from build123d import *

# Parameters (mm, degrees)
SKETCH_1_R               = 246.95
SKETCH_1_R_2             = 223.5
EXTRUDE_5_DEPTH          = 22.45
SKETCH_1_5_R             = 5.6125
CUT_EXTRUDE_1_DEPTH      = 350.960865669
PATTERN_CIRCULAR_2_COUNT = 10


with BuildPart() as part:
    # Эскиз1 → Бобышка-Вытянуть5 (new body)
    with BuildSketch(Plane(origin=(0, 0, 0), x_dir=(1, 0, 0), z_dir=(0, 1, 0))):
        with Locations(Location((0, 0, 0), (0, 0, 270))):
            Circle(SKETCH_1_R)
        with Locations(Location((0, 0, 0), (0, 0, 270))):
            Circle(SKETCH_1_R_2, mode=Mode.SUBTRACT)
    extrude(amount=EXTRUDE_5_DEPTH)

    # Эскиз1<5> → Вырез-Вытянуть1 (cut, through all)
    with BuildSketch(Plane(origin=(0, 0, 0), x_dir=(1, 0, 0), z_dir=(0, 1, 0))):
        with Locations(Location((0, -235.225, 0), (0, 0, 270))):
            Circle(SKETCH_1_5_R)
    cut_extrude_1 = extrude(amount=CUT_EXTRUDE_1_DEPTH, mode=Mode.SUBTRACT)

    # Круговой массив2: Вырез-Вытянуть1 ×10 about axis
    pattern_circular_2_axis = Axis((0, 0, 0), (0, 1, 0))
    for i in range(1, PATTERN_CIRCULAR_2_COUNT):
        add(cut_extrude_1.rotate(pattern_circular_2_axis, i * 360 / PATTERN_CIRCULAR_2_COUNT), mode=Mode.SUBTRACT)


solid = part.part
The listing builds one solid part. Answer for the finished solid, in the listing's coordinates (mm). Coordinates: 2 decimals unless noted, no trailing zeros. Write each loop counter-clockwise with the first axis right and the second up, starting at its lowest first coordinate (ties: lowest second). Pieces come first, ordered by that corner, then holes. Notation, with made-up numbers: (1, 58) - (27, 58) arc R9 ccw to (27, 70) - close; hole circle Ø6 at (16.5, 24.25). An arc over 180 degrees is marked (long way). Return JSON: item names as keys, results as strings.
1. The part is cut by section A-A on z = 0. Determine the outline of the cut face in (x, y), then the cut area to 3 significant figures.
Final values:
{"outline": "(-246.95, 0) - (-223.5, 0) - (-223.5, 22.45) - (-246.95, 22.45) - close; (223.5, 0) - (246.95, 0) - (246.95, 22.45) - (223.5, 22.45) - close", "area": "1,050 mm^2"}
2. The part is cut by section B-B on x = 0. Determine the outline of the cut face in (y, z), then the cut area to 3 significant figures.
Final values:
{"outline": "(0, -246.95) - (22.45, -246.95) - (22.45, -240.84) - (0, -240.84) - close; (0, -229.61) - (22.45, -229.61) - (22.45, -223.5) - (0, -223.5) - close; (0, 223.5) - (22.45, 223.5) - (22.45, 229.61) - (0, 229.61) - close; (0, 240.84) - (22.45, 240.84) - (22.45, 246.95) - (0, 246.95) - close", "area": "549 mm^2"}
3. For a pull along X with two mould halves and no side action, classify faces 1 (the face through (166.901, 11.068, -182.012)), 2 (the face through (1.686, 11.068, 240.578)), 3 (the face through (38, 22.45, -221)), 4 (the face through (-140.045, 11.068, 195.623)) as +X half, -X half, draft (parallel to the pull), parting line (faces both ways), or undercut.
Final values:
{"face 1": "parting line", "face 2": "undercut", "face 3": "draft", "face 4": "undercut"}
4. Each of these flat-tipped pins is pushed along its axis until it touches: pin 1 Ø9 at (x, z) = (0, -235.225) entering from -Y; pin 2 Ø2 at (y, z) = (2.5, -190) entering from -X; pin 3 Ø2 at (y, z) = (15, -180) entering from +X; pin 4 Ø12 at (x, y) = (-82.5, 13.5) entering from +Z. Where does it stop, or does it pass through?
Final values:
{"pin 1": "through", "pin 2": "x = -158.94", "pin 3": "x = 170.13", "pin 4": "z = 234.8"}
5. The part is cut by section D-D on y = 16. Count the separate pieces of the cut face and the enclosed holes in it, then the cut area to 3 significant figures.
Final values:
{"separate pieces": "1", "enclosed holes": "11", "area": "33,700 mm^2"}
6. Consider line 1 along X through (y, z) = (11.25, 195); line 2 along Z through (x, y) = (24, 18.75); line 3 along X through (y, z) = (5.75, 0). Determine where each line is inside the solid, lowest interval first.
Final values:
{"line 1": "-151.52 to -141.33, -135.19 to -109.21, 109.21 to 135.19, 141.33 to 151.52", "line 2": "-245.78 to -222.21, 222.21 to 245.78", "line 3": "-246.95 to -223.5, 223.5 to 246.95"}
7. The part is cut by section C-C on x = 99.5. Determine the outline of the cut face in (y, z), then the cut area to 3 significant figures.
Final values:
{"outline": "(0, -226.02) - (22.45, -226.02) - (22.45, -200.13) - (0, -200.13) - close; (0, 200.13) - (22.45, 200.13) - (22.45, 226.02) - (0, 226.02) - close", "area": "1,160 mm^2"}
